Autodesk Inventor part; units mm, degrees
ref_plane "YZ Plane" through (0, 0, 0) normal (1, 0, 0) x (0, 1, 0)
ref_plane "XZ Plane" through (0, 0, 0) normal (0, 1, 0) x (-1, 0, 0)
ref_plane "XY Plane" through (0, 0, 0) normal (0, 0, 1) x (1, 0, 0)
sketch "Sketch1" plane through (0, 0, 0) normal (0, 1, 0) x (-1, 0, 0)
  circle A0 centre (0, 0) radius 100
  line L0 (0, -140) -> (0, 140)
  line L1 (-146.2506, 0) -> (146.2506, 0)
  circle A1 centre (7.25, 93.75) radius 1.5
  circle A2 centre (-7.25, 93.75) radius 1.5
  circle A3 centre (-44, 60) radius 1.7
  circle A4 centre (-44, -70) radius 1.7
  circle A5 centre (44, 60) radius 1.7
  circle A6 centre (44, -70) radius 1.7
  circle A7 centre (-67, 9) radius 1.25
  circle A8 centre (-67, -9) radius 1.25
  circle A9 centre (67, 9) radius 1.25
  circle A10 centre (67, -9) radius 1.25
  line L2 (-95.8, 24) -> (-73.8, 24)
  line L3 (-73.8, 24) -> (-73.8, -24)
  line L4 (-73.8, -24) -> (-95.8, -24)
  line L5 (-95.8, -24) -> (-95.8, 24)
  line L6 (-95.8, 24) -> (-104.4647, 24)
  line L7 (-104.4647, 24) -> (-104.4647, -24)
  line L8 (-104.4647, -24) -> (-95.8, -24)
  line L9 (-95.8, -24) -> (-95.8, 24)
  line L10 (95.8, 24) -> (73.8, 24)
  line L11 (73.8, 24) -> (73.8, -24)
  line L12 (73.8, -24) -> (95.8, -24)
  line L13 (95.8, -24) -> (95.8, 24)
  line L14 (95.8, 24) -> (104.4647, 24)
  line L15 (104.4647, 24) -> (104.4647, -24)
  line L16 (104.4647, -24) -> (95.8, -24)
  line L17 (95.8, -24) -> (95.8, 24)
  line L18 (-26.5, 78) -> (26.5, 78)
  line L19 (26.5, 78) -> (26.5, 82)
  line L20 (26.5, 82) -> (-26.5, 82)
  line L21 (-26.5, 82) -> (-26.5, 78)
  line L22 (-26.5, 78) -> (-15.9, 78)
  line L23 (-15.9, 78) -> (-15.9, 82)
  line L24 (-15.9, 82) -> (-26.5, 82)
  line L25 (-26.5, 82) -> (-26.5, 78)
  line L26 (-5.3, 78) -> (-5.3, 82)
  line L27 (5.3, 78) -> (5.3, 82)
  line L28 (15.9, 78) -> (15.9, 82)
  line L29 (-26.5, -72) -> (26.5, -72)
  line L30 (26.5, -68) -> (-26.5, -68)
  line L31 (15.9, -72) -> (15.9, -68)
  line L32 (26.5, -72) -> (26.5, -68)
  line L33 (5.3, -72) -> (5.3, -68)
  line L34 (-5.3, -72) -> (-5.3, -68)
  line L35 (-15.9, -72) -> (-15.9, -68)
  line L36 (-26.5, -68) -> (-26.5, -72)
  point P0 (97.0773, 24)
  point P1 (-97.0773, 24)
  point P2 (-97.0773, -24)
  point P3 (97.0773, -24)
  dimension "diam" = 200
  dimension "d3" = 7.25
  dimension "d4" = 7.25
  dimension "d5" = 93.75
  dimension "d6" = 93.75
  dimension "d7" = 3
  dimension "d8" = 3
  dimension "d9" = 60
  dimension "d10" = 3.4
  dimension "d13" = 130
  dimension "d16" = 88
  dimension "d19" = 44
  dimension "d20" = 67
  dimension "d21" = 9
  dimension "d22" = 2.5
  dimension "d25" = 18
  dimension "d28" = 134
  dimension "d31" = 95.8
  dimension "d32" = 24
  dimension "d33" = 22
  dimension "d34" = 48
  dimension "d35" = 78
  dimension "d36" = 26.5
  dimension "d37" = 53
  dimension "d38" = 4
  dimension "d39" = 10.6
  dimension "d40" = 4
  dimension "d43" = 10.6
  dimension "d50" = 150
  dimension "d55" = 0
extrude "Extrusion1" add sketch "Sketch1" along normal blind 4 contours L14 L10 L11 L1 L0 L18 L19 L20 A0 | A0 L0 L29 L32 L30 L1 L11 L12 L16 | L0 L20 L21 L18 L1 L3 L2 L6 A0 | A0 L8 L4 L3 L1 L0 L30 L36 L29 | L20 L28 L18 L27 | L26 L18 L23 L20 | L29 L35 L30 L34 | L33 L30 L31 L29
sketch "Sketch2" plane through (0, 4, 0) normal (0, 1, 0) x (1, 0, 0)
  line L0 (-97.0773, 24) -> (-73.8, 24)
  line L1 (-73.8, 24) -> (-73.8, -24)
  line L2 (-73.8, -24) -> (-97.0773, -24)
  arc A0 (-97.0773, -24) -> (97.0773, -24) centre (0, 0) ccw
  line L3 (97.0773, -24) -> (73.8, -24)
  line L4 (73.8, -24) -> (73.8, 24)
  line L5 (73.8, 24) -> (97.0773, 24)
  arc A1 (97.0773, 24) -> (-97.0773, 24) centre (0, 0) ccw
  line L6 (15.9, -78) -> (26.5, -78)
  line L7 (26.5, -78) -> (26.5, -82)
  line L8 (26.5, -82) -> (15.9, -82)
  line L9 (15.9, -82) -> (15.9, -78)
  line L10 (5.3, 68) -> (-5.3, 68)
  line L11 (-5.3, 68) -> (-5.3, 72)
  line L12 (-5.3, 72) -> (5.3, 72)
  line L13 (5.3, 72) -> (5.3, 68)
  line L14 (15.9, 68) -> (15.9, 72)
  line L15 (15.9, 72) -> (26.5, 72)
  line L16 (26.5, 72) -> (26.5, 68)
  line L17 (26.5, 68) -> (15.9, 68)
  circle A2 centre (67, 9) radius 1.25
  circle A3 centre (44, 70) radius 1.7
  circle A4 centre (-44, 70) radius 1.7
  circle A5 centre (-67, 9) radius 1.25
  line L18 (-15.9, 72) -> (-15.9, 68)
  line L19 (-15.9, 68) -> (-26.5, 68)
  line L20 (-26.5, 68) -> (-26.5, 72)
  line L21 (-26.5, 72) -> (-15.9, 72)
  line L22 (5.3, -78) -> (5.3, -82)
  line L23 (5.3, -82) -> (-5.3, -82)
  line L24 (-5.3, -82) -> (-5.3, -78)
  line L25 (-5.3, -78) -> (5.3, -78)
  circle A6 centre (67, -9) radius 1.25
  circle A7 centre (44, -60) radius 1.7
  circle A8 centre (7.25, -93.75) radius 1.5
  line L26 (-15.9, -78) -> (-15.9, -82)
  line L27 (-15.9, -82) -> (-26.5, -82)
  line L28 (-26.5, -82) -> (-26.5, -78)
  line L29 (-26.5, -78) -> (-15.9, -78)
  circle A9 centre (-67, -9) radius 1.25
  circle A10 centre (-44, -60) radius 1.7
  circle A11 centre (-7.25, -93.75) radius 1.5
equation "\"d19\" = 0.5 * d16"
equation "\"d25\" = 2 * d21"
equation "\"d28\" = 2 * d20"
equation "\"d34\" = 2 * d32"
equation "\"d39\" = 0.2 * d37"
equation "\"d43\" = d39"
equation "\"caster_dist_holes\" = 14.5"
properties part number "base" material "MDF Medium Density Fiberboard"
Verification items for the finished model (mm, model axes). Coordinates: 2 decimals unless noted, no trailing zeros. Loops run counter-clockwise (first coordinate to the right, second up) from the corner with the lowest first, then second, coordinate; pieces in that order, holes last. Notation, with made-up numbers: (60, 8.25) - (117, 8.25) arc R30 ccw to (117, 37.25) - close; hole circle Ø4 at (25, -11.5). An arc over 180 degrees is marked (long way). Put each result on its own line as item: value.
Item 1: Section check A-A (x = 79). Enter the section's corners in (y, z), then the cut area to 3 significant figures.
Conclusion:
outline: (0, -61.31) - (4, -61.31) - (4, -24) - (0, -24) - close; (0, 24) - (4, 24) - (4, 61.31) - (0, 61.31) - close
area: 298 mm2
Item 2: Section check D-D (y = 2.15). Give the number of separate pieces and of enclosed holes in the cut face, then the cut area to 3 significant figures.
Conclusion:
separate pieces: 1
enclosed holes: 16
area: 28,700 mm2
Item 3: Section check C-C (x = 23). Enter the section's corners in (y, z), then the cut area to 3 significant figures.
Conclusion:
outline: (0, -97.32) - (4, -97.32) - (4, -72) - (0, -72) - close; (0, -68) - (4, -68) - (4, 78) - (0, 78) - close; (0, 82) - (4, 82) - (4, 97.32) - (0, 97.32) - close
area: 747 mm2
Item 4: Gauge pin test, flat ends, axial feed: pin 1 Ø1.2 at (x, y) = (-2, 3) entering from -Z; pin 2 Ø1.2 at (x, y) = (-21, 2) entering from +Z; pin 3 Ø2 at (x, y) = (80, 3) entering from -Z. Record the tip position at first contact, or that the pin passes through.
Conclusion:
pin 1: stops at z = -99.99
pin 2: stops at z = 97.9
pin 3: stops at z = -61.31
Item 5: Scan lines: line 1 along Z through (x, y) = (0.5, 3.05); line 2 along Z through (x, y) = (67, 2.2); line 3 along X through (y, z) = (2.2, -70). Record each from-to range of solid material in increasing order.
Conclusion:
line 1: z = -100 to -72, -68 to 78, 82 to 100
line 2: z = -74.24 to -10.25, -7.75 to 7.75, 10.25 to 74.24
line 3: x = -71.41 to -45.7, -42.3 to -26.5, -15.9 to -5.3, 5.3 to 15.9, 26.5 to 42.3, 45.7 to 71.41
Item 6: Section check B-B (z = -3). Enter the section's corners in (x, y).
Conclusion:
outline: (-73.8, 0) - (73.8, 0) - (73.8, 4) - (-73.8, 4) - close
